from build123d import *

# Parameters (mm, degrees)
F0_W = 1
F0_H = 1
F3_R = 0.99999


# Not quite as in the source:
# - a fillet or chamfer is up to 0.001 mm smaller than in the source, because OpenCascade refuses the exact size


with BuildPart() as f1:
    # F0 (on Front) → F1 (revolve)
    with BuildSketch(Plane.XZ):
        Polygon((16, 3.5), (11.2, 3.5), (11.2, 2.5), (11.2, -3.5), (16, -3.5), (12.5, 0), align=None)
        Polygon((10.2, 3.5), (0, 3.5), (0, -3.5), (11.2, -3.5), (11.2, 2.5), (10.2, 2.5), align=None)
        with Locations((10.7, 3)):
            Rectangle(F0_W, F0_H)
    revolve(axis=Axis((0, 0, -0.2485097927), (0, 0, -1)))

    # F0 (on Front) → F2 (revolve, cut)
    with BuildSketch(Plane.XZ):
        Polygon((10.2, 3.5), (0, 3.5), (0, -3.5), (11.2, -3.5), (11.2, 2.5), (10.2, 2.5), align=None)
    revolve(axis=Axis((0, 0, -0.2485097927), (0, 0, -1)), mode=Mode.SUBTRACT)

    # F3 (radius 1 in the source; OpenCascade refuses exactly that, so slightly less here)
    f3_edges = [f1.edges().sort_by_distance(p)[0] for p in [
        (-11.2, 0, 2.5),
    ]]
    fillet(f3_edges, radius=F3_R)


solid = f1.part
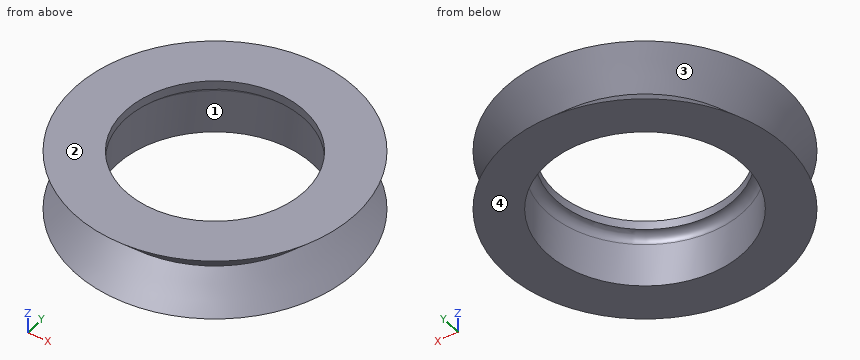
For this review, take the finished solid that the model builds, in its own axes (mm). Face numbers are marked on the shaded views. Coordinates: 2 decimals unless noted, no trailing zeros. Write each question's results on one line, items separated by ' | '.
Q1. Mouldability with a two-part tool opening along Z and no side actions: class the marked faces 1, 2, 3 and 4 as +Z half, -Z half, draft (parallel to the pull), parting line (faces both ways), or undercut.
Taken from the geometry:
face 1: draft | face 2: +Z half | face 3: undercut | face 4: -Z half
Q2. For pin 1 Ø1.5 at (y, z) = (-8, 2.5) entering from +X, flat-tipped, find the tip position at first contact; note if it passes through.
Taken from the geometry:
pin 1: x = 13.67
Q3. To check wall thickness, follow line 1 along X through (y, z) = (-5.5, 0.25); line 2 along X through (y, z) = (0, -1.25); line 3 along Y through (x, z) = (0, 3.15). State the ranges of each line that lie inside material, in increasing order. Write a range as [from, to].
Taken from the geometry:
line 1: [-11.5, -9.76], [9.76, 11.5] | line 2: [-13.75, -11.2], [11.2, 13.75] | line 3: [-15.65, -10.2], [10.2, 15.65]
